from build123d import *

# Parameters (mm, degrees)
F0_W          = 70
F0_H          = 70
F1_DEPTH      = 10
F2_W          = 13
F2_H          = 24.8
F3_DEPTH      = 25
F4_W          = 70
F4_H          = 70
F4_W_2        = 40
F4_H_2        = 40
F5_DEPTH      = 4
F6_W          = 13
F6_H          = 35
F7_DEPTH      = 9
F8_R          = 1.05
F9_DEPTH      = 25
F10_R         = 1.6
F11_DEPTH     = 25
F12_R         = 3.25
F13_DEPTH     = 3
F14_DEPTH     = 4
F15_R         = 34.99999
F16_DEPTH     = 1
F17_T1_DEPTH  = 2e-05
F17_T3_DEPTH  = 2e-05
F17_T6_ANGLE  = 90
F17_T8_ANGLE  = 90
F17_T10_ANGLE = 90
F17_T12_ANGLE = 90


# Not quite as in the source:
# - a fillet or chamfer that OpenCascade refuses, or shapes differently, is made with other operations: its cross-section is extruded or revolved along the edge and cut away or added
# - a fillet or chamfer is up to 0.001 mm smaller than in the source, because OpenCascade refuses the exact size


with BuildPart() as f1:
    # F0 (on Top) → F1 (new body)
    with BuildSketch(Plane.XY):
        Rectangle(F0_W, F0_H)
    extrude(amount=F1_DEPTH)

    # F2 (on face) → F3 (cut)
    with BuildSketch(Plane.XY.offset(10)):
        Rectangle(F2_W, F2_H)
    extrude(amount=-F3_DEPTH, mode=Mode.SUBTRACT)

    # F4 (on face) → F5 (cut)
    with BuildSketch(Plane.XY.offset(10)):
        Rectangle(F4_W, F4_H)
        Rectangle(F4_W_2, F4_H_2, mode=Mode.SUBTRACT)
    extrude(amount=-F5_DEPTH, mode=Mode.SUBTRACT)

    # F6 (on face) → F7 (cut)
    with BuildSketch(Plane.XY.offset(10)):
        Rectangle(F6_W, F6_H)
    extrude(amount=-F7_DEPTH, mode=Mode.SUBTRACT)

    # F8 (on face) → F9 (cut)
    with BuildSketch(Plane.XY.offset(1)):
        with Locations((0, 13.8)):
            Circle(F8_R)
        with Locations((0, -13.8)):
            Circle(F8_R)
    extrude(amount=-F9_DEPTH, mode=Mode.SUBTRACT)

    # F10 (on face) → F11 (cut)
    with BuildSketch(Plane.XY.offset(6)):
        with Locations((-28, 0)):
            Circle(F10_R)
        with Locations((28, 0)):
            Circle(F10_R)
        with Locations((0, -28)):
            Circle(F10_R)
        with Locations((0, 28)):
            Circle(F10_R)
    extrude(amount=-F11_DEPTH, mode=Mode.SUBTRACT)

    # F12 (on face) → F13 (cut)
    with BuildSketch(Plane.XY.offset(6)):
        with Locations((-28, 0)):
            Circle(F12_R)
        with Locations((28, 0)):
            Circle(F12_R)
        with Locations((0, -28)):
            Circle(F12_R)
        with Locations((0, 28)):
            Circle(F12_R)
    extrude(amount=-F13_DEPTH, mode=Mode.SUBTRACT)

    # F14 (cut, through all): a face of the model
    f14_faces = [f1.faces().sort_by_distance(p)[0] for p in [
        (-19.4343145751, 0, 10),
    ]]
    extrude(f14_faces, amount=-F14_DEPTH, mode=Mode.SUBTRACT)

    # F15 (radius 35 in the source; OpenCascade refuses exactly that, so slightly less here)
    f15_edges = [f1.edges().sort_by_distance(p)[0] for p in [
        (-35, -35, 3),
        (35, -35, 3),
        (35, 35, 3),
        (-35, 35, 3),
    ]]
    fillet(f15_edges, radius=F15_R)

    # F16 (add): a face of the model
    f16_faces = [f1.faces().sort_by_distance(p)[0] for p in [
        (0, -34.0100505063, 0),
    ]]
    extrude(f16_faces, amount=F16_DEPTH)

    # F17: fillet of radius 7 on 1 edges, made by hand

    # F17_s2 → F17_t1 (cut)
    with BuildSketch(Plane.YZ.offset(-1e-05)):
        with BuildLine():
            ThreePointArc((-35, -1), (-32.9497474683, 3.9497474683), (-28, 6))
            Line((-28, 6), (-35, 6))
            Line((-35, 6), (-35, -1))
        make_face()
        with BuildLine():
            ThreePointArc((35, -1), (32.9497474683, 3.9497474683), (28, 6))
            Line((28, 6), (35, 6))
            Line((35, 6), (35, -1))
        make_face()
    extrude(amount=F17_T1_DEPTH, mode=Mode.SUBTRACT)

    # F17_s4 → F17_t3 (cut)
    with BuildSketch(Plane.XZ.offset(-1e-05)):
        with BuildLine():
            ThreePointArc((35, -1), (32.9497474683, 3.9497474683), (28, 6))
            Line((28, 6), (35, 6))
            Line((35, 6), (35, -1))
        make_face()
        with BuildLine():
            ThreePointArc((-35, -1), (-32.9497474683, 3.9497474683), (-28, 6))
            Line((-28, 6), (-35, 6))
            Line((-35, 6), (-35, -1))
        make_face()
    extrude(amount=F17_T3_DEPTH, mode=Mode.SUBTRACT)

    # F17_s5 → F17_t6 (revolve, cut)
    with BuildSketch(Plane.YZ.offset(1e-05)):
        with BuildLine():
            ThreePointArc((-35, -1), (-32.9497474683, 3.9497474683), (-28, 6))
            Line((-28, 6), (-35, 6))
            Line((-35, 6), (-35, -1))
        make_face()
    revolve(axis=Axis((1e-05, -1e-05, 6), (0, 0, 1)), revolution_arc=F17_T6_ANGLE, mode=Mode.SUBTRACT)

    # F17_s7 → F17_t8 (revolve, cut)
    with BuildSketch(Plane.XZ.offset(-1e-05)):
        with BuildLine():
            ThreePointArc((35, -1), (32.9497474683, 3.9497474683), (28, 6))
            Line((28, 6), (35, 6))
            Line((35, 6), (35, -1))
        make_face()
    revolve(axis=Axis((1e-05, 1e-05, 6), (0, 0, 1)), revolution_arc=F17_T8_ANGLE, mode=Mode.SUBTRACT)

    # F17_s9 → F17_t10 (revolve, cut)
    with BuildSketch(Plane.XZ.offset(-1e-05)):
        with BuildLine():
            ThreePointArc((-35, -1), (-32.9497474683, 3.9497474683), (-28, 6))
            Line((-28, 6), (-35, 6))
            Line((-35, 6), (-35, -1))
        make_face()
    revolve(axis=Axis((-1e-05, 1e-05, 6), (0, 0, -1)), revolution_arc=F17_T10_ANGLE, mode=Mode.SUBTRACT)

    # F17_s11 → F17_t12 (revolve, cut)
    with BuildSketch(Plane.YZ.offset(-1e-05)):
        with BuildLine():
            ThreePointArc((-28, 6), (-32.9497474683, 3.9497474683), (-35, -1))
            Line((-35, -1), (-35, 6))
            Line((-35, 6), (-28, 6))
        make_face()
    revolve(axis=Axis((-1e-05, -1e-05, 6), (0, 0, -1)), revolution_arc=F17_T12_ANGLE, mode=Mode.SUBTRACT)


solid = f1.part
Can you work these out from the model? Positions are in its coordinate system, mm. A direction names the side the tool comes from. Give positions to 0.01 mm unless a question says otherwise; leave off trailing zeros. Answer as a JSON object with one key per item and string values. Group by question number.
Item 1: For faces 1 (the face through (0, -12.4, 0)), 2 (the face through (-24.9, 0.98, 4.52)), 3 (the face through (7, 0, -1)), which set-ups out of +Z, -Z, +X, -X, +Y, -Y let a thin tool reach every point of the face, with its end or its side?
Item 2: I'm going to push flat-ended pins straight in: P1, Ø5.5, axis at x = 2, y = 14, coming from the +Z side; P2, Ø3.5, axis at x = 28, y = 0, coming from the +Z side; P3, Ø1.5, axis at y = -1, z = 4, coming from the -X side; P4, Ø6, axis at x = 5.5, y = 7.5, coming from the -Z side. Where does each tip first touch, or does it pass through?
Item 3: Please list where these lines run through material, in increasing order: line 1 (Z direction, x = 22, y = 17.5); line 2 (Y direction, x = 0, z = 1.35); line 3 (Y direction, x = -28, z = 0.4). Write a range as [from, to].
Item 4: Suppose I cut it at A-A (z = 2). State how many separate pieces and enclosed holes the cut face has, plus the area to 3 significant figures.
Findings:
{
 "1": {"face 1": "+Z, -Z", "face 2": "+Z", "face 3": "-Z, +X, -X, +Y, -Y"},
 "2": {"P1": "stops at z = 1", "P2": "stops at z = 3", "P3": "stops at x = -33.55", "P4": "stops at z = -1"},
 "3": {"line 1": "z = [-1, 6]", "line 2": "y = [-34.59, -29.6], [-26.4, -17.5], [17.5, 26.4], [29.6, 34.59]", "line 3": "y = [-20.76, -1.6], [1.6, 20.76]"},
 "4": {"separate pieces": "1", "enclosed holes": "5", "area": "3,210 mm²"}
}
